```python
from build123d import *

# Parameters (mm, degrees)
SKETCH1_W           = 80
SKETCH1_H           = 150
BOSS_EXTRUDE1_DEPTH = 27
SKETCH2_W           = 1.5
SKETCH2_H           = 150
CUT_EXTRUDE1_DEPTH  = 24


with BuildPart() as part:
    # Sketch1 → Boss-Extrude1 (new body)
    with BuildSketch(Plane(origin=(0, 0, 0), x_dir=(1, 0, 0), z_dir=(0, 1, 0))):
        with Locations((40, 75)):
            Rectangle(SKETCH1_W, SKETCH1_H)
    extrude(amount=BOSS_EXTRUDE1_DEPTH)

    # Sketch2 → Cut-Extrude1 (cut)
    with BuildSketch(Plane(origin=(0, 27, 0), x_dir=(1, 0, 0), z_dir=(0, 1, 0))):
        with Locations((2.25, 75)):
            Rectangle(SKETCH2_W, SKETCH2_H)
        with Locations((5.395833333, 75)):
            Rectangle(SKETCH2_W, SKETCH2_H)
        with Locations((8.541666667, 75)):
            Rectangle(SKETCH2_W, SKETCH2_H)
        with Locations((11.6875, 75)):
            Rectangle(SKETCH2_W, SKETCH2_H)
        with Locations((14.833333333, 75)):
            Rectangle(SKETCH2_W, SKETCH2_H)
        with Locations((17.979166667, 75)):
            Rectangle(SKETCH2_W, SKETCH2_H)
        with Locations((21.125, 75)):
            Rectangle(SKETCH2_W, SKETCH2_H)
        with Locations((24.270833333, 75)):
            Rectangle(SKETCH2_W, SKETCH2_H)
        with Locations((27.416666667, 75)):
            Rectangle(SKETCH2_W, SKETCH2_H)
        with Locations((30.5625, 75)):
            Rectangle(SKETCH2_W, SKETCH2_H)
        with Locations((33.708333333, 75)):
            Rectangle(SKETCH2_W, SKETCH2_H)
        with Locations((36.854166667, 75)):
            Rectangle(SKETCH2_W, SKETCH2_H)
        with Locations((40, 75)):
            Rectangle(SKETCH2_W, SKETCH2_H)
        with Locations((43.145833333, 75)):
            Rectangle(SKETCH2_W, SKETCH2_H)
        with Locations((46.291666667, 75)):
            Rectangle(SKETCH2_W, SKETCH2_H)
        with Locations((49.4375, 75)):
            Rectangle(SKETCH2_W, SKETCH2_H)
        with Locations((52.583333333, 75)):
            Rectangle(SKETCH2_W, SKETCH2_H)
        with Locations((55.729166667, 75)):
            Rectangle(SKETCH2_W, SKETCH2_H)
        with Locations((58.875, 75)):
            Rectangle(SKETCH2_W, SKETCH2_H)
        with Locations((62.020833333, 75)):
            Rectangle(SKETCH2_W, SKETCH2_H)
        with Locations((65.166666667, 75)):
            Rectangle(SKETCH2_W, SKETCH2_H)
        with Locations((68.3125, 75)):
            Rectangle(SKETCH2_W, SKETCH2_H)
        with Locations((71.458333333, 75)):
            Rectangle(SKETCH2_W, SKETCH2_H)
        with Locations((74.604166667, 75)):
            Rectangle(SKETCH2_W, SKETCH2_H)
        with Locations((77.75, 75)):
            Rectangle(SKETCH2_W, SKETCH2_H)
    extrude(amount=-CUT_EXTRUDE1_DEPTH, mode=Mode.SUBTRACT)


solid = part.part
```
Design review of the part built by this model. Coordinates are the model's own, in mm. A direction names the side the tool comes from. Coordinates: 2 decimals unless noted, no trailing zeros.
1) Mouldability with a two-part tool opening along X and no side actions: class faces 1 (the flat face through (39.25, 15, -74)), 2 (the flat face through (48, 13, 0)), 3 (the flat face through (80, 13, -74)), 4 (the flat face through (37.604, 15, -74)) as +X half, -X half, draft (parallel to the pull), parting line (faces both ways), or undercut.
2) Machinability: for faces 5 (the flat face through (0, 13, -74)), 6 (the flat face through (75.354, 15, -74)), which of the approach directions +Z, -Z, +X, -X, +Y, -Y give a long, thin tool a straight path to every point of the face, cutting with its end or side? Answer none if there is none.
3) Add section A-A (y = 14.75). State how many separate pieces and enclosed holes the cut face has, plus the area to 4 significant figures.
4) To check wall thickness, follow L1, parallel to Y at x = 20.5, z = -133. State the ranges of the line that lie inside material, in increasing order.
5) Insertion check: pin 1 (1.2 mm diameter, centred on x = 62, z = -53, fed in from +Y). The pin has a flat end and moves straight along its axis. Give the tip position at first contact, or say it passes through.
Check result:
1. face 1: undercut
1. face 2: draft
1. face 3: +X half
1. face 4: undercut
2. face 5: +Z, -Z, -X, +Y, -Y
2. face 6: +Z, -Z, +Y
3. separate pieces: 26
3. enclosed holes: 0
3. area: 6,375 mm2
4. L1: y = 0 to 3
5. pin 1: stops at y = 3
